For this review, take the finished solid that the model builds, in its own axes (mm). A direction names the side the tool comes from. Coordinates: 2 decimals unless noted, no trailing zeros. Write each loop counter-clockwise with the first axis right and the second up, starting at its lowest first coordinate (ties: lowest second). Pieces come first, ordered by that corner, then holes. Notation, with made-up numbers: M 87.5,16.5 L 105.5,16.5 A14 cw 105.5,30.5 Z; hole C 31.5,-14 d6. An arc over 180 degrees is marked long. Return JSON: item names as keys, results as strings.
```python
from build123d import *

# Parameters (mm, degrees)
F0_W      = 19.5
F0_H      = 30
F1_DEPTH  = 15
F2_W      = 15.8
F2_H      = 11.45
F3_DEPTH  = 30
F5_DEPTH  = 15
F6_W      = 3.1
F6_H      = 6
F7_DEPTH  = 15
F8_R      = 5
F9_R      = 1
F10_W     = 19.5
F10_H     = 15
F10_W_2   = 16.8
F10_H_2   = 12.45
F11_DEPTH = 5
F12_W     = 16.8
F12_H     = 12.45
F13_DEPTH = 10


with BuildPart() as f1:
    # F0 (on Front) → F1 (new body)
    with BuildSketch(Plane.XZ):
        Rectangle(F0_W, F0_H)
    extrude(amount=F1_DEPTH)

    # F2 (on face) → F3 (cut, through all)
    with BuildSketch(Plane.XY.offset(15)):
        with Locations((0, -7.5)):
            Rectangle(F2_W, F2_H)
    extrude(amount=-F3_DEPTH, mode=Mode.SUBTRACT)

    # F4 (on face) → F5 (join, through all)
    with BuildSketch(Plane.XZ.offset(15)):
        Polygon((-2, 1), (2, 1), (2, 9), (0, 15), (-2, 9), align=None)
    extrude(amount=-F5_DEPTH)

    # F6 (on face) → F7 (cut, through all)
    with BuildSketch(Plane.XZ.offset(15)):
        with Locations((0, 5)):
            Rectangle(F6_W, F6_H)
    extrude(amount=-F7_DEPTH, mode=Mode.SUBTRACT)

    # F8
    f8_edges = [f1.edges().sort_by_distance(p)[0] for p in [
        (-2, -7.5, 9),
        (2, -7.5, 9),
    ]]
    fillet(f8_edges, radius=F8_R)

    # F9
    f9_edges = [f1.edges().sort_by_distance(p)[0] for p in [
        (-2, -7.5, 1),
        (2, -7.5, 1),
    ]]
    fillet(f9_edges, radius=F9_R)

    # F10 (on face) → F11 (cut)
    with BuildSketch(Plane.XY.offset(15)):
        with Locations((0, -7.5)):
            Rectangle(F10_W, F10_H)
        with Locations((0, -7.5)):
            Rectangle(F10_W_2, F10_H_2, mode=Mode.SUBTRACT)
    extrude(amount=-F11_DEPTH, mode=Mode.SUBTRACT)

    # F12 (on face) → F13 (cut)
    with BuildSketch(Plane(origin=(0, 0, -15), x_dir=(1, 0, 0), z_dir=(0, 0, -1))):
        with Locations((0, 7.5)):
            Rectangle(F12_W, F12_H)
    extrude(amount=-F13_DEPTH, mode=Mode.SUBTRACT)


solid = f1.part
```
1. We need section B-B (x = 3.75). State the section outline as (y, z) points (3 decimals).
Checks:
{"outline": "M -15,-15 L -13.725,-15 L -13.725,-5 L -13.225,-5 L -13.225,15 L -13.725,15 L -13.725,10 L -15,10 Z; M -1.775,-5 L -1.275,-5 L -1.275,-15 L 0,-15 L 0,10 L -1.275,10 L -1.275,15 L -1.775,15 Z"}
2. We need section C-C (y = -2.75). Give the number of separate pieces and of enclosed holes in the cut face, plus the area to 3 significant figures.
Checks:
{"separate pieces": "3", "enclosed holes": "1", "area": "112 mm2"}
3. Clearance check with flat-ended pins moving along their axes: pin 1 Ø2.5 at (x, z) = (3, 12.5) entering from -Y (3 decimals); pin 2 Ø2.5 at (y, z) = (-5.5, 12) entering from +X. State where each tip first meets the part, or that it passes through.
Checks:
{"pin 1": "y = -13.725", "pin 2": "x = 8.4"}
4. Draft analysis for pull direction X (two halves, no side actions). For faces 6 (the face through (-9.75, -7, -3)), 7 (the face through (1.699, -7.42, 1.285)), 8 (the face through (0, -1, -15)), 9 (the face through (-8.4, -7, -10)), state which applies: +X half, -X half, draft (parallel to the pull), parting line (faces both ways), or undercut.
Checks:
{"face 6": "-X half", "face 7": "undercut", "face 8": "draft", "face 9": "undercut"}
5. We need section D-D (z = -4.5). State the section outline as (x, y) points (3 decimals).
Checks:
{"outline": "M -9.75,-15 L 9.75,-15 L 9.75,0 L -9.75,0 Z; hole M -7.9,-13.225 L 7.9,-13.225 L 7.9,-1.775 L -7.9,-1.775 Z"}
6. We need section A-A (z = 5.25). State the section outline as (x, y) points (3 decimals), plus the area to 3 significant figures.
Checks:
{"outline": "M -9.75,-15 L -1.55,-15 L -1.55,0 L -9.75,0 Z; M 1.55,-15 L 9.75,-15 L 9.75,0 L 1.55,0 Z; hole M -7.9,-13.225 L -2,-13.225 L -2,-1.775 L -7.9,-1.775 Z; hole M 2,-13.225 L 7.9,-13.225 L 7.9,-1.775 L 2,-1.775 Z", "area": "111 mm2"}
7. For faces 1 (the face through (2, -8, 5)), 2 (the face through (-1.55, -8, 5)), 3 (the face through (0, 0, -2)), 4 (the face through (0, -13.725, -10)), 5 (the face through (1, -8, 12)), list the 3-axis set-ups (+Z, -Z, +X, -X, +Y, -Y) from which the entire face can be reached by the end or side of a thin tool; tool diameter is ignored.
Checks:
{"face 1": "+Z, -Z", "face 2": "+Y, -Y", "face 3": "+Z, -Z, +X, -X, +Y", "face 4": "-Z", "face 5": "+Z"}
8. Wall thickness on L1, parallel to X at y = -4.5, z = 7.25; L2, parallel to Y at x = 3.75, z = -12.5 (3 decimals); L3, parallel to Y at x = -2.75, z = 1.5 (3 decimals): over which ranges is each line inside the solid? List them lowest first. Write a range as from..to.
Checks:
{"L1": "-9.75..-7.9, -2..-1.55, 1.55..2, 7.9..9.75", "L2": "-15..-13.725, -1.275..0", "L3": "-15..-13.225, -1.775..0"}
